Input: dimensioned drawing with shaded views. Units: mm. Origin: part minimum x, y, z. A direction names the side the tool comes from. Coordinates: 2 decimals unless noted, no trailing zeros. Order: outer loops, then holes, each group sorted by start corner. A loop starts at its lowest first (then second) coordinate and runs counter-clockwise, first axis right, second up.
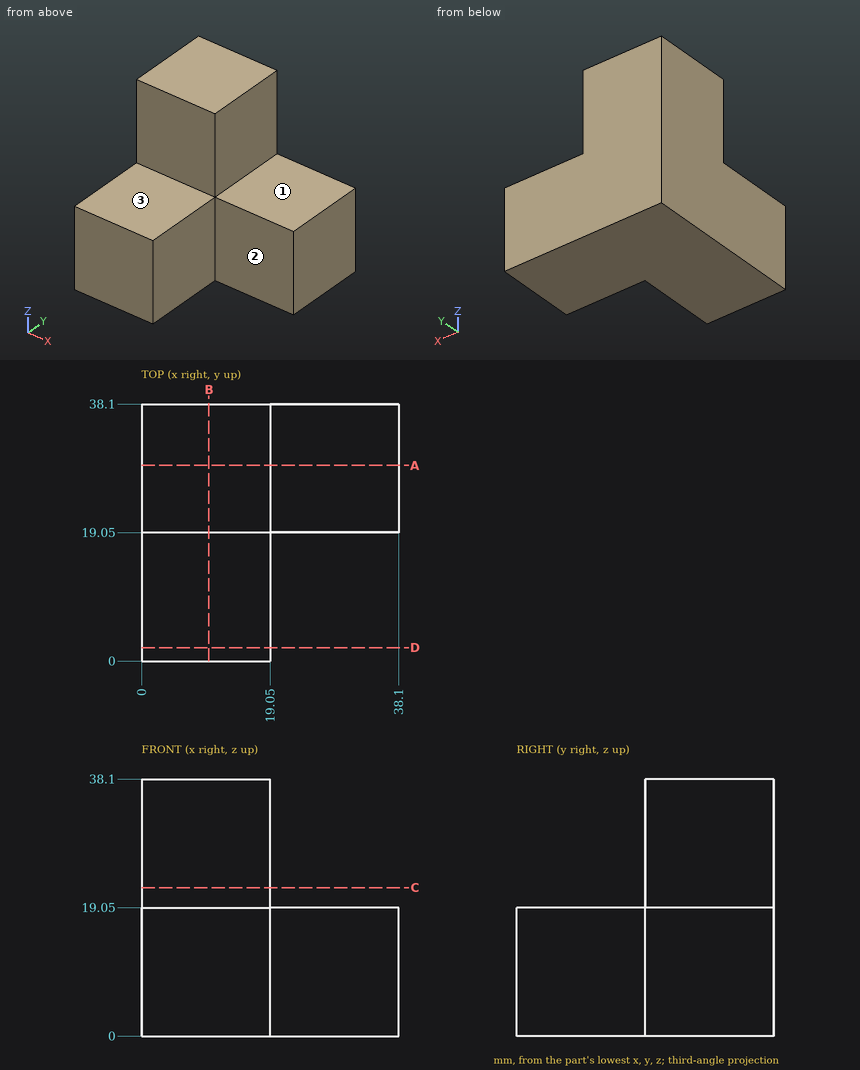
1. Pin query (flat end, axial travel): P1, Ø5.5, axis at x = 32, y = 32, coming from the +Z side; P2, Ø5.5, axis at y = 26.5, z = 24.5, coming from the +X side; P3, Ø15, axis at x = 11, z = 33.5, coming from the -Y side. Return the tip coordinate at first contact, or that it passes through.
Findings:
P1: stops at z = 19.05
P2: stops at x = 19.05
P3: stops at y = 19.05
2. Access query for the marked faces 1, 2 and 3. Directions: +Z, -Z, +X, -X, +Y, -Y. A direction counts if a zero-diameter tool reaches every point of the face in a straight line with its end or side. Return the directions, or none.
Findings:
face 1: +Z, +X, +Y, -Y
face 2: +Z, -Z, +X, -Y
face 3: +Z, +X, -X, -Y
3. Section query B-B on x = 10. Return loops of the section in (y, z).
Findings:
outline: (0, 0) - (38.1, 0) - (38.1, 38.1) - (19.05, 38.1) - (19.05, 19.05) - (0, 19.05) - close
4. Section query A-A on y = 29. Return loops of the section in (x, z).
Findings:
outline: (0, 0) - (38.1, 0) - (38.1, 19.05) - (19.05, 19.05) - (19.05, 38.1) - (0, 38.1) - close
5. Ray query, line 1 (Y direction, x = 21, z = 9); line 2 (X direction, y = 8, z = 5). Return the intervals inside material, ascending.
Findings:
line 1: y = 19.05 to 38.1
line 2: x = 0 to 19.05
6. Section query D-D on y = 2. Return loops of the section in (x, z).
Findings:
outline: (0, 0) - (19.05, 0) - (19.05, 19.05) - (0, 19.05) - close
7. Section query C-C on z = 22. Return loops of the section in (x, y), plus the area to 3 significant figures.
Findings:
outline: (0, 19.05) - (19.05, 19.05) - (19.05, 38.1) - (0, 38.1) - close
area: 363 mm2
